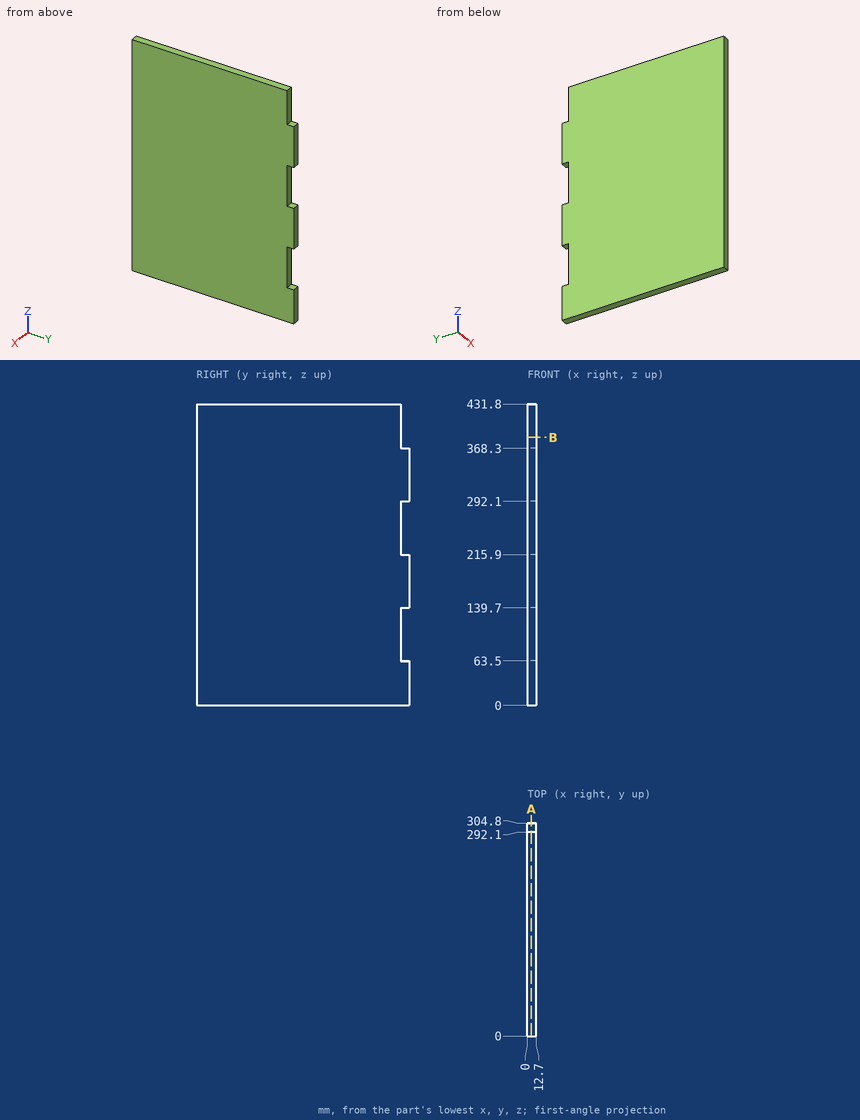
The figure shows three views and two pictorial views of one solid part (mm, origin at its lowest corner). Answer the questions. Give positions to 0.01 mm unless a question says otherwise; leave off trailing zeros. Write each loop counter-clockwise with the first axis right and the second up, starting at its lowest first coordinate (ties: lowest second). Pieces come first, ordered by that corner, then holes. Notation, with made-up numbers: (-14.5, -19) -> (21.5, -19) arc R20 cw to (21.5, -15) -> close; hole circle Ø9 at (65.5, 59). An arc over 180 degrees is marked (long way). Answer as a JSON object with one key per item and string values.
1) A flat-ended cylindrical pin translates along its axis: pin 1 Ø6.5 at (x, z) = (7.5, 386) entering from +Y. Find the tip coordinate at first contact, or state that the pin passes through.
Findings below:
{"pin 1": "stops at y = 292.1"}
2) A straight line is drawn through the part: probe 1 along Y at (x, z) = (9, 77). Find the intervals that lie inside material, in ascending order. Write a range as from..to.
Findings below:
{"probe 1": "y = 0..292.1"}
3) Section A-A on x = 5.75 is taken. Write down the section's boundary in (y, z).
Findings below:
{"outline": "(0, 0) -> (304.8, 0) -> (304.8, 63.5) -> (292.1, 63.5) -> (292.1, 139.7) -> (304.8, 139.7) -> (304.8, 215.9) -> (292.1, 215.9) -> (292.1, 292.1) -> (304.8, 292.1) -> (304.8, 368.3) -> (292.1, 368.3) -> (292.1, 431.8) -> (0, 431.8) -> close"}
4) Section B-B on z = 384 is taken. Write down the section's boundary in (x, y), then the cut area to 3 significant figures.
Findings below:
{"outline": "(0, 0) -> (12.7, 0) -> (12.7, 292.1) -> (0, 292.1) -> close", "area": "3,710 mm^2"}
